Can you work these out from the model? Positions are in its coordinate system, mm. Round coordinates to 2 decimals unless told otherwise and drop trailing zeros. Loops run counter-clockwise (first coordinate to the right, second up) from the corner with the lowest first, then second, coordinate; pieces in that order, holes last. Notation, with made-up numbers: (31.25, 39) -> (82.25, 39) arc R9 cw to (82.25, 46) -> close; hole circle Ø5 at (-40, 5.25). An arc over 180 degrees is marked (long way). Write item = value, one per line.
Autodesk Inventor part; units mm, degrees
ref_plane "YZ Plane" through (0, 0, 0) normal (1, 0, 0) x (0, 1, 0)
ref_plane "XZ Plane" through (0, 0, 0) normal (0, 1, 0) x (-1, 0, 0)
ref_plane "XY Plane" through (0, 0, 0) normal (0, 0, 1) x (1, 0, 0)
sketch "Skizze1" plane through (0, 0, 0) normal (0, 1, 0) x (-1, 0, 0)
  line L0 (-11.455, -18.25) -> (11.455, -18.25)
  line L1 (11.455, -18.25) -> (11.455, 18.25)
  line L2 (11.455, 18.25) -> (-11.455, 18.25)
  line L3 (-11.455, 18.25) -> (-11.455, -18.25)
  line L4 (-11.455, -18.25) -> (11.455, 18.25) construction
  line L5 (11.455, -18.25) -> (-11.455, 18.25) construction
  point P0 (0, 0)
  dimension "d0" = 22.91
  dimension "d1" = 36.5
extrude "Extrusion1" add sketch "Skizze1" along normal blind 1.67
fillet "Rundung1" radius 2.5 4 edges at (-11.455, 0.835, 18.25) (11.455, 0.835, -18.25) (11.455, 0.835, 18.25) (-11.455, 0.835, -18.25)
sketch "Skizze2" plane through (0, 1.67, 0) normal (0, 1, 0) x (1, 0, 0)
  circle A0 centre (-8.955, -15.75) radius 1.3
  line L0 (-8.955, -18.25) -> (8.955, -18.25)
  line L1 (-11.455, 15.75) -> (-11.455, -15.75)
  line L2 (0, 0) -> (0, -21.9467) construction
  circle A1 centre (8.955, -15.75) radius 1.3
  dimension "d5" = 2.6
  dimension "d6" = 2.5
  dimension "d7" = 2.5
  dimension "d8" = 17.91
extrude "Extrusion2" cut sketch "Skizze2" against normal up to next
properties part number "PowerBoost500"
1. Suppose I cut it at A-A, the plane y = 0.85. List the corners of the cut face in (x, z) for me (3 decimals), and give its area (3 significant figures).
Entries:
outline = (-11.455, -15.75) arc R2.5 ccw to (-8.955, -18.25) -> (8.955, -18.25) arc R2.5 ccw to (11.455, -15.75) -> (11.455, 15.75) arc R2.5 ccw to (8.955, 18.25) -> (-8.955, 18.25) arc R2.5 ccw to (-11.455, 15.75) -> close; hole circle Ø2.6 at (-8.955, 15.75); hole circle Ø2.6 at (8.955, 15.75)
area = 820 mm²
2. I need wall thicknesses on line 1 (X direction, y = 1.3, z = 15.75) (3 decimals); line 2 (Z direction, x = -8.5, y = 1.3); line 3 (Z direction, x = 9.75, y = 1.1). Which ranges of each line are inside material? Lowest first, please. Write a range as [from, to].
Entries:
line_1 = [-11.455, -10.255], [-7.655, 7.655], [10.255, 11.455]
line_2 = [-18.25, 14.53], [16.97, 18.25]
line_3 = [-18.12, 14.72], [16.78, 18.12]
3. We'd pull the mould along X, two halves only. Please class faces 1 (the flat face through (11.455, 1, 0)), 2 (the cylindrical face through (-8.26, 0.85, 14.65)), 3 (the flat face through (0, 0, 0)): released by +X, released by -X, zero draft, split by the parting line, or undercut.
Entries:
face_1 = released by +X
face_2 = undercut
face_3 = zero draft
